Could you check a few things on this drawing? It's one solid part, dimensions in mm from its lowest x, y, z. A direction names the side the tool comes from. Coordinates: 2 decimals unless noted, no trailing zeros. Loops run counter-clockwise (first coordinate to the right, second up) from the corner with the lowest first, then second, coordinate; pieces in that order, holes last. Notation, with made-up numbers: M -10,66.5 L 26,66.5 A12 cw 26,79.5 Z; hole C 50,60.5 d3. An arc over 180 degrees is marked long. Use one line per item in the form item = value. Start each with the question number.
(1) On a 3-axis mill with a long thin cutter (end or side, diameter ignored), from which of +Z, -Z, +X, -X, +Y, -Y can I reach the whole of each face in a straight line? I mean the marked faces 1, 2, 3 and 4. Say none if no direction works.
(2) Will these pins go through, and if not, where does the flat tip stop? P1, Ø1, axis at x = 71.5, z = 1, coming from the +Y side; P2, Ø1, axis at y = 58.5, z = 1, coming from the -X side; P3, Ø3, axis at x = 83.5, z = 3, coming from the +Y side; P4, Ø8, axis at x = 59, z = 17, coming from the +Y side.
(3) Please list where this line runs through material, in increasing order: L1, parallel to Y at x = 47.5, z = 14.25.
(4) Imagine slicing it at A-A, the plane x = 87. Please give me the cut outline in (y, z), and give its area (3 significant figures).
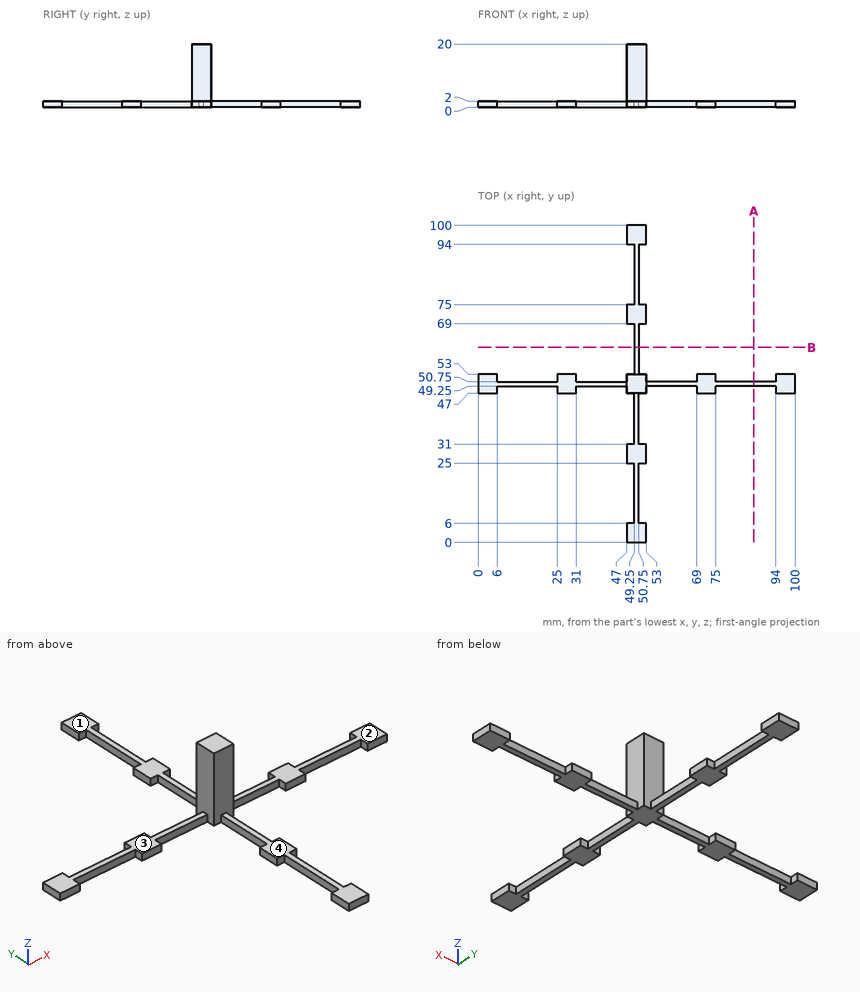
Answer:
q1.face_1 = +Z, +X, -X, +Y
q1.face_2 = +Z, +X, +Y, -Y
q1.face_3 = +Z, -X, +Y, -Y
q1.face_4 = +Z, +X, -X, -Y
q2.P1 = 53
q2.P2 = 49.25
q2.P3 = 50.75
q2.P4 = through
q3.L1 = 47 to 53
q4.outline = M 49.25,0 L 50.75,0 L 50.75,2 L 49.25,2 Z
q4.area = 3.00 mm²
